from build123d import *

# Parameters (mm, degrees)
SKETCH1_W           = 101
SKETCH1_H           = 95
BOSS_EXTRUDE1_DEPTH = 1.2
SKETCH3_W           = 101
SKETCH3_H           = 95
SKETCH3_W_2         = 96
SKETCH3_H_2         = 90
BOSS_EXTRUDE2_DEPTH = 5
SKETCH5_R           = 3
BOSS_EXTRUDE3_DEPTH = 3.2
CUT_EXTRUDE1_REACH  = 6.4
SKETCH6_R           = 1.7
CUT_EXTRUDE2_REACH  = 3.2
SKETCH7_W           = 22
SKETCH7_H           = 10
FILLET1_R           = 3
SKETCH8_W           = 97
SKETCH8_H           = 91
SKETCH8_W_2         = 96
SKETCH8_H_2         = 90
BOSS_EXTRUDE4_DEPTH = 1.5


with BuildPart() as part:
    # Sketch1 → Boss-Extrude1 (new body)
    with BuildSketch(Plane(origin=(0, 0, 0), x_dir=(1, 0, 0), z_dir=(0, 1, 0))):
        with Locations((46.5, 43.5)):
            Rectangle(SKETCH1_W, SKETCH1_H)
    extrude(amount=BOSS_EXTRUDE1_DEPTH)

    # Sketch3 → Boss-Extrude2 (add)
    with BuildSketch(Plane(origin=(0, 1.2, 0), x_dir=(1, 0, 0), z_dir=(0, 1, 0))):
        with Locations((46.5, 43.5)):
            Rectangle(SKETCH3_W, SKETCH3_H)
        with Locations((46.5, 43.5)):
            Rectangle(SKETCH3_W_2, SKETCH3_H_2, mode=Mode.SUBTRACT)
    extrude(amount=BOSS_EXTRUDE2_DEPTH)

    # Sketch5 → Boss-Extrude3 (add)
    with BuildSketch(Plane(origin=(0, 1.2, 0), x_dir=(1, 0, 0), z_dir=(0, 1, 0))):
        with Locations((2.5, 84.5)):
            Circle(SKETCH5_R)
        with Locations((90.5, 84.5)):
            Circle(SKETCH5_R)
        with Locations((90.5, 19.5)):
            Circle(SKETCH5_R)
        with Locations((2.5, 19.5)):
            Circle(SKETCH5_R)
    extrude(amount=BOSS_EXTRUDE3_DEPTH)

    # Sketch6 → Cut-Extrude1 (cut, up to next)
    with BuildSketch(Plane(origin=(0, 4.4, 0), x_dir=(1, 0, 0), z_dir=(0, 1, 0)), mode=Mode.PRIVATE) as cut_extrude1_sk1:
        with Locations((2.5, 84.5)):
            Circle(SKETCH6_R)
    cut_extrude1_tool1 = extrude(cut_extrude1_sk1.sketch, amount=-CUT_EXTRUDE1_REACH, mode=Mode.PRIVATE) & part.part
    add(cut_extrude1_tool1.solids().sort_by_distance((2.5, 4.4, -84.5))[0], mode=Mode.SUBTRACT)
    # Sketch6 → Cut-Extrude1 (cut, up to next)
    with BuildSketch(Plane(origin=(0, 4.4, 0), x_dir=(1, 0, 0), z_dir=(0, 1, 0)), mode=Mode.PRIVATE) as cut_extrude1_sk2:
        with Locations((90.5, 84.5)):
            Circle(SKETCH6_R)
    cut_extrude1_tool2 = extrude(cut_extrude1_sk2.sketch, amount=-CUT_EXTRUDE1_REACH, mode=Mode.PRIVATE) & part.part
    add(cut_extrude1_tool2.solids().sort_by_distance((90.5, 4.4, -84.5))[0], mode=Mode.SUBTRACT)
    # Sketch6 → Cut-Extrude1 (cut, up to next)
    with BuildSketch(Plane(origin=(0, 4.4, 0), x_dir=(1, 0, 0), z_dir=(0, 1, 0)), mode=Mode.PRIVATE) as cut_extrude1_sk3:
        with Locations((90.5, 19.5)):
            Circle(SKETCH6_R)
    cut_extrude1_tool3 = extrude(cut_extrude1_sk3.sketch, amount=-CUT_EXTRUDE1_REACH, mode=Mode.PRIVATE) & part.part
    add(cut_extrude1_tool3.solids().sort_by_distance((90.5, 4.4, -19.5))[0], mode=Mode.SUBTRACT)
    # Sketch6 → Cut-Extrude1 (cut, up to next)
    with BuildSketch(Plane(origin=(0, 4.4, 0), x_dir=(1, 0, 0), z_dir=(0, 1, 0)), mode=Mode.PRIVATE) as cut_extrude1_sk4:
        with Locations((2.5, 19.5)):
            Circle(SKETCH6_R)
    cut_extrude1_tool4 = extrude(cut_extrude1_sk4.sketch, amount=-CUT_EXTRUDE1_REACH, mode=Mode.PRIVATE) & part.part
    add(cut_extrude1_tool4.solids().sort_by_distance((2.5, 4.4, -19.5))[0], mode=Mode.SUBTRACT)

    # Sketch7 → Cut-Extrude2 (cut, up to next)
    with BuildSketch(Plane(origin=(0, 1.2, 0), x_dir=(1, 0, 0), z_dir=(0, 1, 0)), mode=Mode.PRIVATE) as cut_extrude2_sk1:
        with Locations((61.5, 76)):
            Rectangle(SKETCH7_W, SKETCH7_H)
    cut_extrude2_tool1 = extrude(cut_extrude2_sk1.sketch, amount=-CUT_EXTRUDE2_REACH, mode=Mode.PRIVATE) & part.part
    add(cut_extrude2_tool1.solids().sort_by_distance((61.5, 1.2, -76))[0], mode=Mode.SUBTRACT)
    # Sketch7 → Cut-Extrude2 (cut, up to next)
    with BuildSketch(Plane(origin=(0, 1.2, 0), x_dir=(1, 0, 0), z_dir=(0, 1, 0)), mode=Mode.PRIVATE) as cut_extrude2_sk2:
        with Locations((31.5, 76)):
            Rectangle(SKETCH7_W, SKETCH7_H)
    cut_extrude2_tool2 = extrude(cut_extrude2_sk2.sketch, amount=-CUT_EXTRUDE2_REACH, mode=Mode.PRIVATE) & part.part
    add(cut_extrude2_tool2.solids().sort_by_distance((31.5, 1.2, -76))[0], mode=Mode.SUBTRACT)

    # Fillet1
    fillet1_edges = [part.edges().sort_by_distance(p)[0] for p in [
        (-4, 3.1, -91),
        (97, 3.1, -91),
        (97, 3.1, 4),
        (-4, 3.1, 4),
    ]]
    fillet(fillet1_edges, radius=FILLET1_R)

    # Sketch8 → Boss-Extrude4 (add)
    with BuildSketch(Plane(origin=(0, 6.2, 0), x_dir=(1, 0, 0), z_dir=(0, 1, 0))):
        with Locations((46.5, 43.5)):
            Rectangle(SKETCH8_W, SKETCH8_H)
        with Locations((46.5, 43.5)):
            Rectangle(SKETCH8_W_2, SKETCH8_H_2, mode=Mode.SUBTRACT)
    extrude(amount=BOSS_EXTRUDE4_DEPTH)


solid = part.part
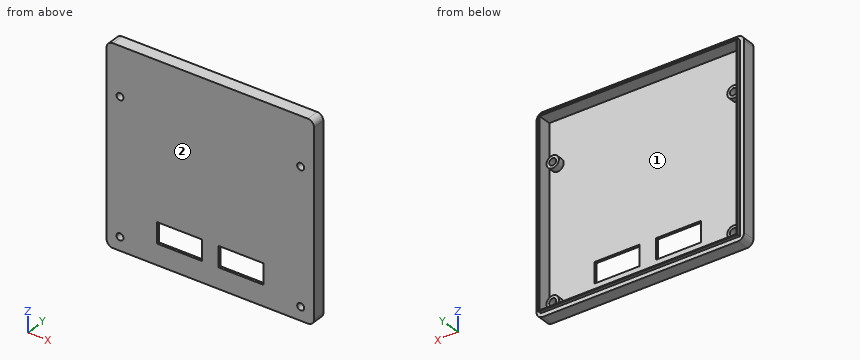
Check sheet for the modelled part. Datum: model origin and axes. Units: mm. Face numbers are marked on the shaded views. Give positions to 0.01 mm unless a question says otherwise; leave off trailing zeros. Loops run counter-clockwise (first coordinate to the right, second up) from the corner with the lowest first, then second, coordinate; pieces in that order, holes last. Notation, with made-up numbers: M 51,72 L 104,72 A19 cw 104,79 Z; hole C 54,-36.75 d3. An arc over 180 degrees is marked long. Use a Markdown table: item, result. Add a question column.
Q1. Sectioned sample at B-B, the plane z = -84.5. Record the cut outline in (x, y).
Q2. Mould release check, pull along Z, two halves, no side actions. Record for the marked faces 1 and 2: pulls with the +Z half, pulls with the -Z half, needs draft (parallel to the pull), parting line crosses it, or undercut.
Q3. Scan lines: line 1 along Z through (x, y) = (90.5, 2.65); line 2 along X through (y, z) = (2.2, -84.5); line 3 along X through (y, z) = (1, -72). Record each from-to range of solid material in increasing order. Write a range as [from, to].
Q4. Go/stop test with a flat-tipped pin: pin 1 (6 mm diameter, centred on x = 58, z = -61.5, fed in from +Y). Record where the tip stops, or that it passes through.
Q5. Sectioned sample at D-D, the plane x = 90.5. Record the cut outline in (y, z), then the cut area to 3 significant figures.
Q6. Sectioned sample at A-A, the plane y = 3. Give the number of separate pieces and of enclosed holes in the cut face, then the cut area to 3 significant figures.
Q7. Sectioned sample at C-C, the plane x = 60.5. Record the cut outline in (y, z), then the cut area to 4 significant figures.
Verdict:
| question | item | result |
|---|---|---|
| 1 | outline | M -4,0 L 0.8,0 L 0.8,4.4 L -0.5,4.4 L -0.5,1.2 L -1.5,1.2 L -1.5,7.7 L -2,7.7 L -2,6.2 L -4,6.2 Z; M 4.2,0 L 88.8,0 L 88.8,4.4 L 87.5,4.4 L 87.5,1.2 L 5.5,1.2 L 5.5,4.4 L 4.2,4.4 Z; M 92.2,0 L 97,0 L 97,6.2 L 95,6.2 L 95,7.7 L 94.5,7.7 L 94.5,1.2 L 93.5,1.2 L 93.5,4.4 L 92.2,4.4 Z |
| 2 | face 1 | undercut |
| 2 | face 2 | needs draft |
| 3 | line 1 | [-91, -88.5], [-87.5, -86.2], [-82.8, -81.5], [-22.5, -21.2], [-17.8, -16.5], [1.5, 4] |
| 3 | line 2 | [-4, -1.5], [-0.5, 0.8], [4.2, 5.5], [87.5, 88.8], [92.2, 93.5], [94.5, 97] |
| 3 | line 3 | [-4, 20.5], [42.5, 50.5], [72.5, 97] |
| 4 | pin 1 | y = 1.2 |
| 5 | outline | M 0,-91 L 6.2,-91 L 6.2,-89 L 7.7,-89 L 7.7,-88.5 L 1.2,-88.5 L 1.2,-87.5 L 4.4,-87.5 L 4.4,-86.2 L 0,-86.2 Z; M 0,-82.8 L 4.4,-82.8 L 4.4,-81.5 L 1.2,-81.5 L 1.2,-22.5 L 4.4,-22.5 L 4.4,-21.2 L 0,-21.2 Z; M 0,-17.8 L 4.4,-17.8 L 4.4,-16.5 L 1.2,-16.5 L 1.2,1.5 L 7.7,1.5 L 7.7,2 L 6.2,2 L 6.2,4 L 0,4 Z |
| 5 | area | 149 mm^2 |
| 6 | separate pieces | 5 |
| 6 | enclosed holes | 5 |
| 6 | area | 1,020 mm^2 |
| 7 | outline | M 0,-91 L 6.2,-91 L 6.2,-89 L 7.7,-89 L 7.7,-88.5 L 1.2,-88.5 L 1.2,-81 L 0,-81 Z; M 0,-71 L 1.2,-71 L 1.2,1.5 L 7.7,1.5 L 7.7,2 L 6.2,2 L 6.2,4 L 0,4 Z |
| 7 | area | 128.5 mm^2 |
